Can you work these out from the model? Positions are in its coordinate system, mm. A direction names the side the tool comes from. Coordinates: 2 decimals unless noted, no trailing zeros. Order: outer loops, then holes, each group sorted by start corner. A loop starts at its lowest first (then second) coordinate and runs counter-clockwise, first axis right, second up. Notation, with made-up numbers: (25.25, 2) - (45.25, 2) arc R31 cw to (45.25, 32) - close; hole circle Ø10 at (-29.75, 6.25). An arc over 180 degrees is marked (long way). Use a Markdown table: item, result. Add a question column.
(1) I want a section at C-C (x = 6). List the corners of the cut face in (y, z) for me.
(2) I want a section at A-A (x = -11). List the corners of the cut face in (y, z) for me, and give its area (3 significant figures).
(3) We'd pull the mould along Y, two halves only. Please class faces 1 (the flat face through (0, -50, 5)), 2 (the cylindrical face through (-10.84, 43.24, 4.93)), 3 (the flat face through (0, 50, 5)): pulls with the +Y half, pulls with the -Y half, needs draft (parallel to the pull), parting line crosses it, or undercut.
(4) I want a section at D-D (y = -42). List the corners of the cut face in (x, z) for me, and give its area (3 significant figures).
(5) On a 3-axis mill with a long thin cutter (end or side, diameter ignored), from which of +Z, -Z, +X, -X, +Y, -Y can I reach the whole of each face in a straight line? I mean faces 4 (the cylindrical face through (-17.2, 46.24, 5.16)), 5 (the cylindrical face through (14.25, -41.95, 4.93)). Say none if no direction works.
(6) For pin 1 Ø2 at (y, z) = (45, 5) entering from -X, with a flat end and sliding along its axis, tell me the tip position at first contact or that it passes through.
(7) If I drill on L1, parallel to Y at x = -16.5, z = 5; L2, parallel to Y at x = 6, z = 4.25; L3, parallel to Y at x = -11.5, z = 2.25, over which ranges is the centre line in solid material (lowest first)? Write a range as [from, to].
(8) I want a section at B-B (y = -12). List the corners of the cut face in (x, z) for me, and give its area (3 significant figures).
```python
from build123d import *

# Parameters (mm, degrees)
SKETCH1_W                      = 42
SKETCH1_H                      = 100
BOSS_EXTRUDE1_DEPTH            = 10
F_12_0_12_DIAMETER_HOLE1_D     = 12
F_2_5_2_5_DIAMETER_HOLE1_D     = 2.5
F_2_5_2_5_DIAMETER_HOLE2_D     = 2.5
F_2_5_2_5_DIAMETER_HOLE2_DEPTH = 7.5
F_2_5_2_5_DIAMETER_HOLE2_TIP   = 0.751075774


with BuildPart() as part:
    # Sketch1 → Boss-Extrude1 (new body)
    with BuildSketch(Plane.XY.offset(10)):
        Rectangle(SKETCH1_W, SKETCH1_H)
    extrude(amount=-BOSS_EXTRUDE1_DEPTH)

    # Ø12.0 (12) Diameter Hole1 (through all)
    with Locations(Plane(origin=(0, 0, 0), x_dir=(-1, 0, 0), z_dir=(0, 0, -1))):
        with Locations((-6, -12)):
            Hole(F_12_0_12_DIAMETER_HOLE1_D / 2)

    # Ø2.5 (2.5) Diameter Hole1 (through all)
    with Locations(Plane.XY.offset(10)):
        with Locations((13, 42), (-11, 42), (-11, -42), (13, -42)):
            Hole(F_2_5_2_5_DIAMETER_HOLE1_D / 2)

    # Ø2.5 (2.5) Diameter Hole2
    with Locations(Plane.ZY.offset(21)):
        with Locations((5, 45), (5, -45)):
            Hole(F_2_5_2_5_DIAMETER_HOLE2_D / 2, depth=F_2_5_2_5_DIAMETER_HOLE2_DEPTH)
            with Locations((0, 0, -(F_2_5_2_5_DIAMETER_HOLE2_DEPTH + F_2_5_2_5_DIAMETER_HOLE2_TIP / 2))):  # 118° drill point
                Cone(0, F_2_5_2_5_DIAMETER_HOLE2_D / 2, F_2_5_2_5_DIAMETER_HOLE2_TIP, mode=Mode.SUBTRACT)


solid = part.part
```
Answers follow:
| question | item | result |
|---|---|---|
| 1 | outline | (-50, 0) - (-18, 0) - (-18, 10) - (-50, 10) - close; (-6, 0) - (50, 0) - (50, 10) - (-6, 10) - close |
| 2 | outline | (-50, 0) - (-43.25, 0) - (-43.25, 10) - (-50, 10) - close; (-40.75, 0) - (40.75, 0) - (40.75, 10) - (-40.75, 10) - close; (43.25, 0) - (50, 0) - (50, 10) - (43.25, 10) - close |
| 2 | area | 950 mm² |
| 3 | face 1 | pulls with the -Y half |
| 3 | face 2 | undercut |
| 3 | face 3 | pulls with the +Y half |
| 4 | outline | (-21, 0) - (-12.25, 0) - (-12.25, 10) - (-21, 10) - close; (-9.75, 0) - (11.75, 0) - (11.75, 10) - (-9.75, 10) - close; (14.25, 0) - (21, 0) - (21, 10) - (14.25, 10) - close |
| 4 | area | 370 mm² |
| 5 | face 4 | -X |
| 5 | face 5 | +Z, -Z |
| 6 | pin 1 | stops at x = -13.35 |
| 7 | L1 | y = [-50, -46.25], [-43.75, 43.75], [46.25, 50] |
| 7 | L2 | y = [-50, -18], [-6, 50] |
| 7 | L3 | y = [-50, -43.15], [-40.85, 40.85], [43.15, 50] |
| 8 | outline | (-21, 0) - (0, 0) - (0, 10) - (-21, 10) - close; (12, 0) - (21, 0) - (21, 10) - (12, 10) - close |
| 8 | area | 300 mm² |
